The model under review builds one solid part; all positions refer to its coordinate system, in mm. Give positions to 0.01 mm unless a question says otherwise; leave off trailing zeros. Write item = value, one per line.
```python
from build123d import *

# Parameters (mm, degrees)
SKETCH1_W            = 72
SKETCH1_H            = 56
BOSS_EXTRUDE1_DEPTH  = 2
SKETCH2_R            = 2
CUT_EXTRUDE1_DEPTH   = 3
LPATTERN1_COUNT      = 9
LPATTERN1_PITCH      = 8
LPATTERN1_COUNT_DIR2 = 7
LPATTERN1_PITCH_DIR2 = 8
SKETCH4_R            = 4
CUT_EXTRUDE2_DEPTH   = 3
LPATTERN2_COUNT      = 4
LPATTERN2_PITCH      = 16
LPATTERN2_COUNT_DIR2 = 3
LPATTERN2_PITCH_DIR2 = 16
FILLET1_R            = 4


with BuildPart() as part:
    # Sketch1 → Boss-Extrude1 (new body)
    with BuildSketch(Plane.XY):
        Rectangle(SKETCH1_W, SKETCH1_H)
    extrude(amount=BOSS_EXTRUDE1_DEPTH)

    # Sketch2 → Cut-Extrude1 (cut)
    with BuildSketch(Plane.XY.offset(2)):
        with Locations((-32, 24)):
            Circle(SKETCH2_R)
    cut_extrude1 = extrude(amount=-CUT_EXTRUDE1_DEPTH, mode=Mode.SUBTRACT)

    # LPattern1: Cut-Extrude1 9 × 7
    with Locations(*[(i * LPATTERN1_PITCH, -j * LPATTERN1_PITCH_DIR2, 0) for i in range(LPATTERN1_COUNT) for j in range(LPATTERN1_COUNT_DIR2) if (i, j) != (0, 0)]):
        add(cut_extrude1, mode=Mode.SUBTRACT)

    # Sketch4 → Cut-Extrude2 (cut)
    with BuildSketch(Plane.XY.offset(2)):
        with Locations((-24, 16)):
            Circle(SKETCH4_R)
    cut_extrude2 = extrude(amount=-CUT_EXTRUDE2_DEPTH, mode=Mode.SUBTRACT)

    # LPattern2: Cut-Extrude2 4 × 3
    with Locations(*[(i * LPATTERN2_PITCH, -j * LPATTERN2_PITCH_DIR2, 0) for i in range(LPATTERN2_COUNT) for j in range(LPATTERN2_COUNT_DIR2) if (i, j) != (0, 0)]):
        add(cut_extrude2, mode=Mode.SUBTRACT)

    # Fillet1
    fillet1_edges = [part.edges().sort_by_distance(p)[0] for p in [
        (36, -28, 1),
        (-36, -28, 1),
        (-36, 28, 1),
        (36, 28, 1),
    ]]
    fillet(fillet1_edges, radius=FILLET1_R)


solid = part.part
```
1. Take a section at A-A on x = -24. Count the separate pieces of the cut face and the enclosed holes in it, and give its area (3 significant figures).
Findings below:
separate_pieces = 8
enclosed_holes = 0
area = 32.0 mm²
2. For line 1 (Y direction, x = 20.5, z = 0.7); line 2 (X direction, y = 3, z = 1.8); line 3 (X direction, y = 12.5, z = 0.1), list the stretches that pass through material, from the lowest coordinate up. Write a range as from..to.
Findings below:
line_1 = -28..-17.94, -14.06..-1.94, 1.94..14.06, 17.94..28
line_2 = -36..-26.65, -21.35..-10.65, -5.35..5.35, 10.65..21.35, 26.65..36
line_3 = -36..-25.94, -22.06..-9.94, -6.06..6.06, 9.94..22.06, 25.94..36
3. Draft analysis for pull direction Y (two halves, no side actions). For faces 1 (the flat face through (-36, 0, 1)), 2 (the cylindrical face through (7.479, 19.966, 1.014)), state which applies: +Y half, -Y half, draft (parallel to the pull), parting line (faces both ways), or undercut.
Findings below:
face_1 = draft
face_2 = undercut
